Print and shaded views of the part. All mm, measured from the part's lowest x, y and z. A direction names the side the tool comes from. Round coordinates to 2 decimals unless told otherwise and drop trailing zeros. Order: outer loops, then holes, each group sorted by start corner. A loop starts at its lowest first (then second) coordinate and runs counter-clockwise, first axis right, second up.
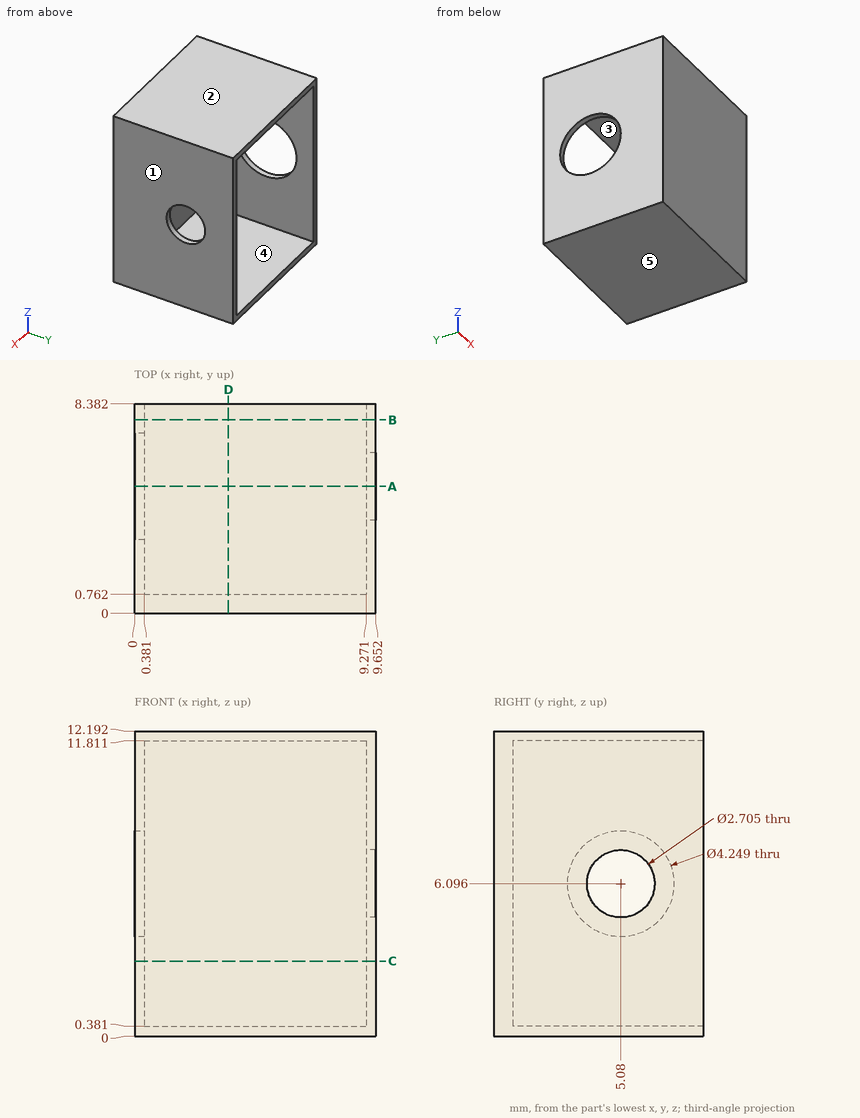
1. Cut at C-C, the plane z = 3. Write the cut outline in (x, y).
2. Drill centre lines: line 1 (Z direction, x = 1.25, y = 4); line 2 (X direction, y = 2.5, z = 3); line 3 (Y direction, x = 7, z = 8.5). Where is each one in solid material? Low to high.
3. Cut at B-B, the plane y = 7.75. Write the cut outline in (x, z).
4. Mould opens along Z. For the marked faces 1, 2 and 3 say: released by +Z, released by -Z, zero draft, split by the parting line, or undercut.
5. Cut at A-A, the plane y = 5.08. Write the cut outline in (x, z).
6. Tool access for the marked faces 4 and 5: list every direction of +Z, -Z, +X, -X, +Y, -Y with a clear straight run to the whole face (end or side of a thin tool).
7. Cut at D-D, the plane x = 3.75. Write the cut outline in (y, z).
Outcome:
1. outline: (0, 0) - (9.65, 0) - (9.65, 8.38) - (9.27, 8.38) - (9.27, 0.76) - (0.38, 0.76) - (0.38, 8.38) - (0, 8.38) - close
2. line 1: z = 0 to 0.38, 11.81 to 12.19
2. line 2: x = 0 to 0.38, 9.27 to 9.65
2. line 3: y = 0 to 0.76
3. outline: (0, 0) - (9.65, 0) - (9.65, 12.19) - (0, 12.19) - close; hole (0.38, 0.38) - (9.27, 0.38) - (9.27, 11.81) - (0.38, 11.81) - close
4. face 1: zero draft
4. face 2: released by +Z
4. face 3: undercut
5. outline: (0, 0) - (9.65, 0) - (9.65, 4.74) - (9.27, 4.74) - (9.27, 0.38) - (0.38, 0.38) - (0.38, 3.97) - (0, 3.97) - close; (0, 8.22) - (0.38, 8.22) - (0.38, 11.81) - (9.27, 11.81) - (9.27, 7.45) - (9.65, 7.45) - (9.65, 12.19) - (0, 12.19) - close
6. face 4: +Y
6. face 5: -Z, +X, -X, +Y, -Y
7. outline: (0, 0) - (8.38, 0) - (8.38, 0.38) - (0.76, 0.38) - (0.76, 11.81) - (8.38, 11.81) - (8.38, 12.19) - (0, 12.19) - close
